Autodesk Fusion 360 part; units mm, degrees
sketch "base sketch" plane through (0, 0, 0) normal (0, 0, 1) x (1, 0, 0)
  line L0 (-44, 15.5) -> (44, 15.5)
  line L1 (44, 15.5) -> (44, -15.5)
  line L2 (44, -15.5) -> (-44, -15.5)
  line L3 (-44, -15.5) -> (-44, 15.5)
  line L4 (-44, 15.5) -> (-44, 34.3701)
  line L5 (44, 15.5) -> (44, 34.3701)
  line L6 (-26.8701, 51.5) -> (26.8701, 51.5)
  line L7 (0, -15.5) -> (0, 51.5)
  line L8 (-19, -12.5) -> (-19, -15.5)
  line L9 (19, -12.5) -> (19, -15.5)
  line L10 (-19, -12.5) -> (19, -12.5)
  line L11 (-5, -12.5) -> (-5, -8.5)
  line L12 (5, -12.5) -> (5, -8.5)
  line L13 (-5, -8.5) -> (5, -8.5)
  circle A0 centre (-25, 15.5) radius 5
  circle A1 centre (25, 15.5) radius 5
  circle A2 centre (0, 51.5) radius 19
  line L14 (0, 51.5) -> (13.435, 64.935)
  line L15 (0, 51.5) -> (19, 51.5) construction
  line L16 (0, 51.5) -> (-13.435, 64.935)
  line L17 (-13.435, 64.935) -> (-44, 34.3701)
  line L18 (13.435, 64.935) -> (44, 34.3701)
  line L19 (-44, -15.5) -> (44, -15.5)
  line L20 (44, -15.5) -> (44, -28.5)
  line L21 (-44, -28.5) -> (-44, -15.5)
  circle A3 centre (0, -34.5) radius 9.5
  circle A4 centre (0, -34.5) radius 19
  line L22 (44, -28.5) -> (18.0278, -28.5)
  line L23 (-18.0278, -28.5) -> (-44, -28.5)
  line L24 (-44, -28.5) -> (-18.0278, -28.5)
  line L25 (18.0278, -28.5) -> (44, -28.5)
  dimension "d2" = 31
  dimension "d10" = 38
  dimension "d11" = 25
  dimension "d12" = 4
  dimension "d13" = 4
  dimension "d14" = 39
  dimension "d15" = 10
  dimension "d16" = 10
  dimension "d17" = 10
  dimension "d18" = 50
  dimension "d19" = 19
  dimension "d20" = 38
  dimension "d21" = 45
  dimension "d27" = 13
  dimension "d30" = 19
  dimension "d31" = 38
extrude "Extrude1" add sketch "base sketch" along normal blind 10 contours L0 L5 L6 L7 A1 A2 L18 | L0 L1 L2 L7 L9 L10 L12 L13 A1 L19 | L0 L2 L3 L7 L8 L10 L11 L13 A0 L19 | L0 L4 L6 L7 A0 A2 L17 | L6 A2 L18 | L6 L7 A2 | L6 L7 A2 | L6 A2 L14 | A2 L14 L16 | L6 A2 L16 | L6 A2 L17 makes body 1
extrude "Extrude2" add sketch "base sketch" along normal blind 50 contours L2 L19 L20 A4 L22 L25 | L2 L7 L9 L10 L19 | L7 L10 L12 L13 | L7 L10 L11 L13 | L2 L19 L21 A4 L23 L24 | L2 L7 L8 L10 L19 | A4 bodies 1
fillet "Fillet1" radius 13 1 edges at (44, 34.3701, 5) on bodies 1
fillet "Fillet2" radius 13 1 edges at (-44, 34.3701, 5) on bodies 1
fillet "Fillet3" radius 3 1 edges at (-19, -15.5, 30) on bodies 1
fillet "Fillet4" radius 3 1 edges at (19, -15.5, 30) on bodies 1
fillet "Fillet5" radius 6 1 edges at (18.0278, -28.5, 25) on bodies 1
fillet "Fillet6" radius 6 1 edges at (-18.0278, -28.5, 25) on bodies 1
sketch "slope sketch" plane through (0, 0, 0) normal (1, 0, 0) x (0, 1, 0)
  line L0 (-8.5, 0) -> (51.5, 0)
  line L1 (-8.5, 0) -> (-8.5, 10)
  line L2 (-8.5, 10) -> (51.5, 10)
  line L3 (51.5, 10) -> (51.5, 0)
  line L4 (-8.5, 10) -> (-8.5, 50)
  line L5 (-8.5, 50) -> (51.5, 10)
  dimension "d48" = 60
  dimension "d49" = 40
extrude "Extrude3" add sketch "slope sketch" along normal mid plane 10 contours L2 L4 L5 bodies 1
copy_body "Body->Comp1" bodies 1 removing the originals makes body 2 in component "object A3"
component "object A3" placed x (1, 0, 0) y (0, 1, 0) z (0, 0, 1) at (0, 0, 0)
Read the model definition and answer for the solid it produces. Units are mm, in the model's axes. A direction names the side the tool comes from. Coordinates: 2 decimals unless noted, no trailing zeros. Loops run counter-clockwise (first coordinate to the right, second up) from the corner with the lowest first, then second, coordinate; pieces in that order, holes last.
(1) Flat-ended cylindrical pins translate along their axes: pin 1 Ø6 at (x, y) = (15, 46) entering from -Z; pin 2 Ø1.5 at (x, y) = (34.5, -30) entering from -Z; pin 3 Ø13 at (x, y) = (25, 15.5) entering from +Z; pin 4 Ø9.5 at (x, z) = (34, 21) entering from -Y. Find the tip coordinate at first contact, or state that the pin passes through.
Solution:
pin 1: stops at z = 0
pin 2: passes through
pin 3: stops at z = 10
pin 4: stops at y = -28.5
(2) The part is cut by section C-C (y = 15.5). Determine the outline of the cut face in (x, z), and give its area (3 significant figures).
Solution:
outline: (-44, 0) - (-30, 0) - (-30, 10) - (-44, 10) - close; (-20, 0) - (20, 0) - (20, 10) - (5, 10) - (5, 34) - (-5, 34) - (-5, 10) - (-20, 10) - close; (30, 0) - (44, 0) - (44, 10) - (30, 10) - close
area: 920 mm2
(3) The part is cut by section A-A (x = 0). Determine the outline of the cut face in (y, z).
Solution:
outline: (-53.5, 0) - (-44, 0) - (-44, 50) - (-53.5, 50) - close; (-25, 0) - (70.5, 0) - (70.5, 10) - (51.5, 10) - (-8.5, 50) - (-25, 50) - close
(4) The mould has two halves that part along X. Classify faces 6 (the face through (-19.9, -14.64, 30.28)), 7 (the face through (43.04, 33.89, 5.07)), 8 (the face through (12, -12.5, 30)), 9 (the face through (21, 18.5, 4.9)): released by +X, released by -X, zero draft, split by the parting line, or undercut.
Solution:
face 6: released by -X
face 7: released by +X
face 8: zero draft
face 9: undercut
(5) A tool of negligible diameter and unlimited length cuts with its end or side. For faces 1 (the face through (35, -28.5, 25)), 2 (the face through (5, 12, 25)), 3 (the face through (-1, -21, 50)), 4 (the face through (-34, -28.5, 25)), 5 (the face through (-5, 12, 25)), from which of +Z, -Z, +X, -X, +Y, -Y can it reach the whole face along a straight path? Write none if from no direction.
Solution:
face 1: +Z, -Z, +X, -Y
face 2: +Z, +X, +Y
face 3: +Z, +X, -X, +Y, -Y
face 4: +Z, -Z, -X, -Y
face 5: +Z, -X, +Y
(6) Consider line 1 along X through (y, z) = (15.5, 5.5); line 2 along Z through (x, y) = (-31, 2); line 3 along Y through (x, z) = (-26, 19). Determine where each line is inside the solid, lowest interval first.
Solution:
line 1: x = -44 to -30, -20 to 20, 30 to 44
line 2: z = 0 to 10
line 3: y = -28.5 to -15.5
